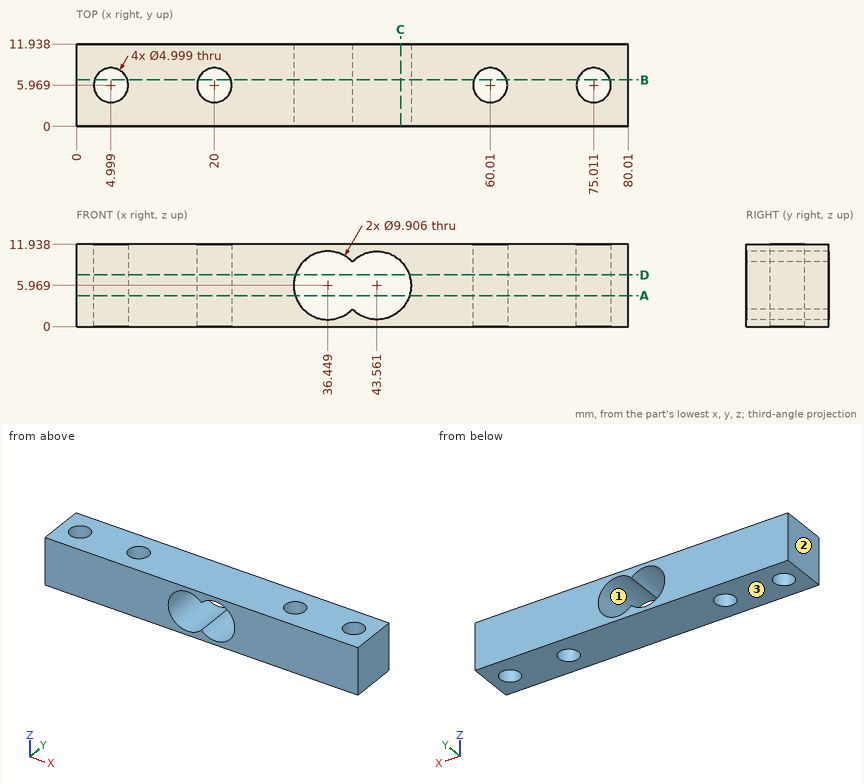
Design review of the part shown in the three views and the two pictorial views. Dimensions are in mm from the part's minimum x, y and z. Give positions to 0.01 mm unless a question says otherwise; leave off trailing zeros. Loops run counter-clockwise (first coordinate to the right, second up) from the corner with the lowest first, then second, coordinate; pieces in that order, holes last. Notation, with made-up numbers: (4.5, 41.5) - (45.5, 41.5) arc R26 cw to (45.5, 58.5) - close; hole circle Ø7 at (-22, 51.5). An arc over 180 degrees is marked (long way). Answer as a JSON object with one key per item and string values.
Q1. Add section A-A on z = 4.5. State the section outline as (x, y) points.
Worked out:
{"outline": "(0, 0) - (31.72, 0) - (31.72, 11.94) - (0, 11.94) - close; (48.29, 0) - (80.01, 0) - (80.01, 11.94) - (48.29, 11.94) - close; hole circle Ø5 at (5, 5.97); hole circle Ø5 at (20, 5.97); hole circle Ø5 at (60.01, 5.97); hole circle Ø5 at (75.01, 5.97)"}
Q2. Insertion check: pin 1 (6 mm diameter, centred on x = 36.449, z = 5.969, fed in from -Y). The pin has a flat end and moves straight along its axis. Give the tip position at first contact, or say it passes through.
Worked out:
{"pin 1": "passes through"}
Q3. To check wall thickness, follow line 1 along X through (y, z) = (5.75, 8.75); line 2 along X through (y, z) = (9.25, 7.5); line 3 along Y through (x, z) = (73.5, 1). State the ranges of each line that lie inside material, in increasing order.
Worked out:
{"line 1": "x = 0 to 2.51, 7.49 to 17.51, 22.49 to 32.35, 47.66 to 57.52, 62.5 to 72.52, 77.5 to 80.01", "line 2": "x = 0 to 31.74, 48.27 to 80.01", "line 3": "y = 0 to 3.98, 7.96 to 11.94"}
Q4. Add section C-C on x = 47. State the section outline as (y, z) points (1 decimal).
Worked out:
{"outline": "(0, 0) - (11.9, 0) - (11.9, 2.4) - (0, 2.4) - close; (0, 9.5) - (11.9, 9.5) - (11.9, 11.9) - (0, 11.9) - close"}
Q5. Mouldability with a two-part tool opening along Z and no side actions: class the marked faces 1, 2 and 3 as +Z half, -Z half, draft (parallel to the pull), parting line (faces both ways), or undercut.
Worked out:
{"face 1": "undercut", "face 2": "draft", "face 3": "-Z half"}
Q6. Add section B-B on y = 6.75. State the section outline as (x, z) points (1 decimal).
Worked out:
{"outline": "(0, 0) - (2.6, 0) - (2.6, 11.9) - (0, 11.9) - close; (7.4, 0) - (17.6, 0) - (17.6, 11.9) - (7.4, 11.9) - close; (22.4, 0) - (57.6, 0) - (57.6, 11.9) - (22.4, 11.9) - close; (62.4, 0) - (72.6, 0) - (72.6, 11.9) - (62.4, 11.9) - close; (77.4, 0) - (80, 0) - (80, 11.9) - (77.4, 11.9) - close; hole (40, 2.5) arc R5 ccw (long way) to (40, 9.4) arc R5 ccw (long way) to start"}
Q7. Add section D-D on z = 7.5. State the section outline as (x, y) points, plus the area to 3 significant figures.
Worked out:
{"outline": "(0, 0) - (31.74, 0) - (31.74, 11.94) - (0, 11.94) - close; (48.27, 0) - (80.01, 0) - (80.01, 11.94) - (48.27, 11.94) - close; hole circle Ø5 at (5, 5.97); hole circle Ø5 at (20, 5.97); hole circle Ø5 at (60.01, 5.97); hole circle Ø5 at (75.01, 5.97)", "area": "679 mm^2"}
